Geometry check sheet. Reference: drawing and pictorial views, mm from the part's lowest x, y, z. Round coordinates to 2 decimals unless told otherwise and drop trailing zeros. Order: outer loops, then holes, each group sorted by start corner. A loop starts at its lowest first (then second) coordinate and runs counter-clockwise, first axis right, second up.
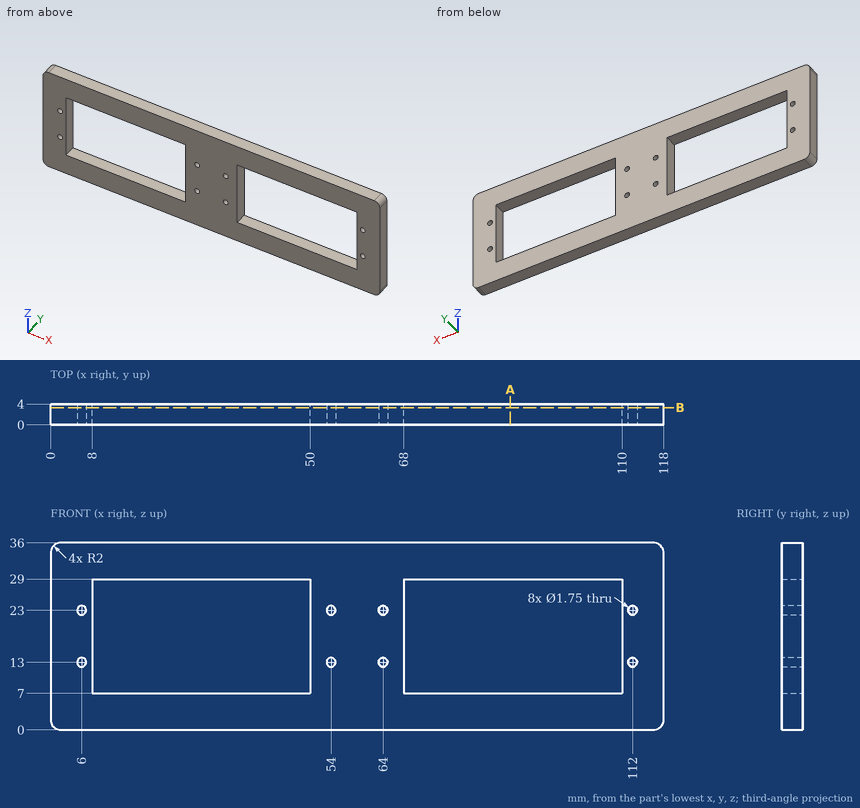
1) Scan lines: probe 1 along Z at (x, y) = (64, 2.3) (3 decimals); probe 2 along X at (y, z) = (1.85, 12); probe 3 along Z at (x, y) = (49, 1.8). Record each from-to range of solid material in increasing order.
2) Sectioned sample at B-B on y = 3.3. Count the separate pieces of the cut face and the enclosed holes in it, then the cut area to 3 significant figures.
3) Sectioned sample at A-A on x = 88.5. Record the cut outline in (y, z).
Returned:
1. probe 1: z = 0 to 12.125, 13.875 to 22.125, 23.875 to 36
1. probe 2: x = 0 to 8, 50 to 68, 110 to 118
1. probe 3: z = 0 to 7, 29 to 36
2. separate pieces: 1
2. enclosed holes: 10
2. area: 2,380 mm2
3. outline: (0, 0) - (4, 0) - (4, 7) - (0, 7) - close; (0, 29) - (4, 29) - (4, 36) - (0, 36) - close
